from build123d import *

# Parameters (mm, degrees)
SKETCH1_W               = 40.5
SKETCH1_H               = 20.5
BOSS_EXTRUDE1_DEPTH     = 3.5
SKETCH2_R               = 1.55
SKETCH2_W               = 3.5
SKETCH2_H               = 6
CUT_EXTRUDE1_DEPTH      = 50.747487374
SKETCH3_W               = 15
SKETCH3_H               = 3.5
CUT_EXTRUDE2_DEPTH      = 50.747487374
CUT_EXTRUDE3_DEPTH      = 50.747487374
CUT_EXTRUDE3_DEPTH_BACK = 50.747487374
SKETCH4_R               = 1.5
CUT_EXTRUDE4_REACH      = 51.747
SKETCH5_R               = 1.55
SKETCH6_W               = 30
SKETCH6_H               = 3
CUT_EXTRUDE5_DEPTH      = 10


with BuildPart() as part:
    # Sketch1 → Boss-Extrude1 (new body)
    with BuildSketch(Plane.XY):
        with BuildLine():
            Line((-35.75, -31), (35.75, -31))
            ThreePointArc((35.75, -31), (37.871320344, -30.121320344), (38.75, -28))
            Line((38.75, -28), (38.75, 28))
            ThreePointArc((38.75, 28), (37.871320344, 30.121320344), (35.75, 31))
            Line((35.75, 31), (-35.75, 31))
            ThreePointArc((-35.75, 31), (-37.871320344, 30.121320344), (-38.75, 28))
            Line((-38.75, 28), (-38.75, -28))
            ThreePointArc((-38.75, -28), (-37.871320344, -30.121320344), (-35.75, -31))
        make_face()
        with Locations((-9.5, 14.75)):
            Rectangle(SKETCH1_W, SKETCH1_H, mode=Mode.SUBTRACT)
    extrude(amount=BOSS_EXTRUDE1_DEPTH)

    # Sketch2 → Cut-Extrude1 (cut, through all)
    with BuildSketch(Plane.XY.offset(3.5)):
        with Locations((33.75, -19.5)):
            Circle(SKETCH2_R)
        with Locations(Location((-33.75, -19.5, 0), (0, 0, 180))):
            Circle(SKETCH2_R)
        with Locations((33.75, -13)):
            Rectangle(SKETCH2_W, SKETCH2_H)
        with Locations((33.75, -26)):
            Rectangle(SKETCH2_W, SKETCH2_H)
        with Locations((-33.75, -26)):
            Rectangle(SKETCH2_W, SKETCH2_H)
        with Locations((-33.75, -13)):
            Rectangle(SKETCH2_W, SKETCH2_H)
    extrude(amount=-CUT_EXTRUDE1_DEPTH, mode=Mode.SUBTRACT)

    # Sketch3 → Cut-Extrude2 (cut, through all)
    with BuildSketch(Plane.XY.offset(3.5)):
        with Locations((-19.75, -24.75)):
            Rectangle(SKETCH3_W, SKETCH3_H)
        with Locations((19.75, -24.75)):
            Rectangle(SKETCH3_W, SKETCH3_H)
    extrude(amount=-CUT_EXTRUDE2_DEPTH, mode=Mode.SUBTRACT)

    # Sketch4 → Cut-Extrude3 (cut, two sides: drawn at the far end of the back side and taken through both)
    with BuildSketch(Plane.XY.offset(3.5).offset(-CUT_EXTRUDE3_DEPTH_BACK)):
        with Locations((15, 19.5)):
            Circle(SKETCH4_R)
        with Locations((15, 10)):
            Circle(SKETCH4_R)
        with Locations((-34, 10)):
            Circle(SKETCH4_R)
        with Locations((-34, 19.5)):
            Circle(SKETCH4_R)
    extrude(amount=CUT_EXTRUDE3_DEPTH + CUT_EXTRUDE3_DEPTH_BACK, mode=Mode.SUBTRACT)

    # Sketch5 → Cut-Extrude4 (cut, up to next)
    with BuildSketch(Plane.XY.offset(3.5), mode=Mode.PRIVATE) as cut_extrude4_sk1:
        with Locations((-34, 0.5)):
            Circle(SKETCH5_R)
    cut_extrude4_tool1 = extrude(cut_extrude4_sk1.sketch, amount=-CUT_EXTRUDE4_REACH, mode=Mode.PRIVATE) & part.part
    add(cut_extrude4_tool1.solids().sort_by_distance((-34, 0.5, 3.5))[0], mode=Mode.SUBTRACT)

    # Sketch6 → Cut-Extrude5 (cut)
    with BuildSketch(Plane.XY.offset(3.5)):
        with Locations((0, -29.5)):
            Rectangle(SKETCH6_W, SKETCH6_H)
    extrude(amount=-CUT_EXTRUDE5_DEPTH, mode=Mode.SUBTRACT)


solid = part.part
Source: CAD feature listing. Evaluate the final solid. Frame: model axes, mm. A direction names the side the tool comes from. Coordinates: 2 decimals unless noted, no trailing zeros. Order: outer loops, then holes, each group sorted by start corner. A loop starts at its lowest first (then second) coordinate and runs counter-clockwise, first axis right, second up. Notation, with made-up numbers: M -21,82.25 L -2,82.25 A24 cw -2,106.25 Z; hole C 72,5.5 d6. An arc over 180 degrees is marked long. Write each question's results on one line, items separated by ' | '. Start each with the question number.
Item 1: Draft query along X for faces 3 (the face through (-26, -31, 2)), 4 (the face through (-35.2, 9.1, 1.7)), 5 (the face through (-37.85, 30.14, 1.73)). Return one class per face: pulls with the +X half, pulls with the -X half, needs draft (parallel to the pull), parting line crosses it, or undercut.
Item 2: Cut plane D-D (y = -25.5). Return loops of the section in (x, z).
Item 3: Cut plane C-C (x = 6). Return loops of the section in (y, z), and give its area (3 significant figures).
Item 4: Cut plane B-B (x = -21.5). Return loops of the section in (y, z), and give its area (3 significant figures).
Item 5: Cut plane A-A (y = 19.5). Return loops of the section in (x, z), and give its area (4 significant figures).
Item 6: Line query: probe 1 along X at (y, z) = (10, 2.55); probe 2 along Y at (x, z) = (34, 2.9); probe 3 along Y at (x, z) = (-15.5, 0.8). Output: solid intervals per line, ascending.
Item 7: Set-up query: faces 1 (the face through (38.75, 0, 2)), 2 (the face through (-27.25, -25, 2)). Return all of +Z, -Z, +X, -X, +Y, -Y with unobstructed straight access to the full face (end or side cutting, diameter ignored); none if empty.
Checked values:
1) face 3: needs draft | face 4: undercut | face 5: pulls with the -X half
2) outline: M -38.75,0 L -35.5,0 L -35.5,3.5 L -38.75,3.5 Z; M -32,0 L -27.25,0 L -27.25,3.5 L -32,3.5 Z; M -12.25,0 L 12.25,0 L 12.25,3.5 L -12.25,3.5 Z; M 27.25,0 L 32,0 L 32,3.5 L 27.25,3.5 Z; M 35.5,0 L 38.75,0 L 38.75,3.5 L 35.5,3.5 Z
3) outline: M -28,0 L 4.5,0 L 4.5,3.5 L -28,3.5 Z; M 25,0 L 31,0 L 31,3.5 L 25,3.5 Z | area: 135 mm2
4) outline: M -31,0 L -26.5,0 L -26.5,3.5 L -31,3.5 Z; M -23,0 L 4.5,0 L 4.5,3.5 L -23,3.5 Z; M 25,0 L 31,0 L 31,3.5 L 25,3.5 Z | area: 133 mm2
5) outline: M -38.75,0 L -35.5,0 L -35.5,3.5 L -38.75,3.5 Z; M -32.5,0 L -29.75,0 L -29.75,3.5 L -32.5,3.5 Z; M 10.75,0 L 13.5,0 L 13.5,3.5 L 10.75,3.5 Z; M 16.5,0 L 38.75,0 L 38.75,3.5 L 16.5,3.5 Z | area: 108.5 mm2
6) probe 1: x = -38.75 to -35.5, -32.5 to -29.75, 10.75 to 13.5, 16.5 to 38.75 | probe 2: y = -31 to -29, -23 to -21.03, -17.97 to -16, -10 to 31 | probe 3: y = -31 to -26.5, -23 to 4.5, 25 to 31
7) face 1: +Z, -Z, +X, +Y, -Y | face 2: +Z, -Z
